Could you check a few things on this model? Use its own coordinates, in mm. A direction names the side the tool comes from. Give positions to 0.01 mm unless a question says otherwise; leave off trailing zeros. Order: outer loops, then holes, each group sorted by start corner. A loop starts at its lowest first (then second) coordinate and runs counter-clockwise, first axis right, second up.
(1) If we mould it in two halves opening along Y, with no side actions, what happens to faces 1 (the flat face through (165.2, -25.6, 67.4)), 2 (the flat face through (107.5, -25, 105)), 3 (the flat face through (142, -150, 82))? For each: released by +Y, released by -Y, zero draft, split by the parting line, or undercut.
(2) Imagine slicing it at D-D, the plane y = -124. Write out the boundary of the cut face in (x, z), then the cut area to 3 significant figures.
(3) Imagine slicing it at A-A, the plane x = 170.5. Write out the boundary of the cut face in (y, z).
(4) On a 3-axis mill with a long thin cutter (end or side, diameter ignored), from which of +Z, -Z, +X, -X, +Y, -Y can I reach the whole of each face in a straight line? I mean faces 4 (the flat face through (99, -60, 20)), 5 (the flat face through (99, 10, 20)), 6 (the flat face through (180, -26, 40)), 7 (the flat face through (65, -26, 83)). Say none if no direction works.
(5) Imagine slicing it at B-B, the plane y = -25. Write out the boundary of the cut face in (x, z).
(6) If I drill on probe 1 along X at (y, z) = (-64.5, 88); probe 2 along Y at (x, z) = (105, 112); probe 3 along Y at (x, z) = (28, 22), over which ranges is the centre line in solid material (lowest first)?
(7) Will these pins go through, and if not, where does the flat tip stop? pin 1 (10 mm diameter, centred on x = 134, z = 11.5, fed in from -Y); pin 2 (2 mm diameter, centred on x = 78.5, z = 69.5, fed in from -Y); pin 3 (12 mm diameter, centred on x = 152, z = 61, fed in from +Y); pin 4 (22 mm diameter, centred on x = 83.5, y = 8.5, fed in from -Z).
(8) Imagine slicing it at C-C, the plane z = 96.5. Write out the boundary of the cut face in (x, y).
from build123d import *

# Parameters (mm, degrees)
SKETCH_1_W          = 200
SKETCH_1_H          = 50
EXTRUDE_1_DEPTH     = 20
SKETCH_2_W          = 160
SKETCH_2_H          = 90
EXTRUDE_2_DEPTH     = 40
SKETCH_3_W          = 15
SKETCH_3_H          = 15
EXTRUDE_3_DEPTH     = 90
EXTRUDE_START       = -45
SKETCH_5_W          = 15
SKETCH_5_H          = 15
EXTRUDE_4_DEPTH     = 125
SKETCH_6_R          = 30
EXTRUDE_5_DEPTH     = 30
SKETCH_7_W          = 30
SKETCH_7_H          = 5
CUT_EXTRUDE_2_DEPTH = 30


with BuildPart() as part:
    # Эскиз1 → Бобышка-Вытянуть1 (new body)
    with BuildSketch(Plane.XY):
        with Locations((100, -25)):
            Rectangle(SKETCH_1_W, SKETCH_1_H)
    extrude(amount=EXTRUDE_1_DEPTH)

    # Эскиз2 → Бобышка-Вытянуть2 (add)
    with BuildSketch(Plane.XY.offset(20)):
        with Locations((100, -25)):
            Rectangle(SKETCH_2_W, SKETCH_2_H)
    extrude(amount=EXTRUDE_2_DEPTH)

    # Эскиз3 → Бобышка-Вытянуть3 (add)
    with BuildSketch(Plane.XZ.offset(70)):
        Polygon((65, 90), (65, 75), (65, 60), (135, 60), (135, 75), (135, 90), align=None)
        with Locations((142.5, 82.5)):
            Rectangle(SKETCH_3_W, SKETCH_3_H)
        Polygon((135, 75), (135, 60), (180, 60), (150, 75), align=None)
        Polygon((65, 75), (20, 60), (65, 60), align=None)
    extrude(amount=-EXTRUDE_3_DEPTH)

    # Эскиз5 → Бобышка-Вытянуть4 (add, symmetric)
    with BuildSketch(Plane(origin=(0, 20, 0), x_dir=(1, 0, 0), z_dir=(0, 1, 0)).offset(EXTRUDE_START)):
        with Locations((142.5, -82.5)):
            Rectangle(SKETCH_5_W, SKETCH_5_H)
    extrude(amount=EXTRUDE_4_DEPTH, both=True)

    # Эскиз6 → Бобышка-Вытянуть5 (add)
    with BuildSketch(Plane.XY.offset(90)):
        with Locations((107.5, -25)):
            Circle(SKETCH_6_R)
    extrude(amount=EXTRUDE_5_DEPTH)

    # Эскиз7 → Вырез-Вытянуть2 (cut)
    with BuildSketch(Plane.XY.offset(120)):
        with Locations((92.5, -27.5)):
            Rectangle(SKETCH_7_W, SKETCH_7_H)
        with Locations((92.5, -22.5)):
            Rectangle(SKETCH_7_W, SKETCH_7_H)
    extrude(amount=-CUT_EXTRUDE_2_DEPTH, mode=Mode.SUBTRACT)


solid = part.part
Answer block:
1. face 1: zero draft
1. face 2: undercut
1. face 3: released by -Y
2. outline: (135, 75) - (150, 75) - (150, 90) - (135, 90) - close
2. area: 225 mm2
3. outline: (-70, 20) - (-50, 20) - (-50, 0) - (0, 0) - (0, 20) - (20, 20) - (20, 64.75) - (-70, 64.75) - close
4. face 4: -Z, +X, -X, -Y
4. face 5: -Z, +X, -X, +Y
4. face 6: +Z, +X, +Y, -Y
4. face 7: +Z, -X, +Y, -Y
5. outline: (0, 0) - (200, 0) - (200, 20) - (180, 20) - (180, 60) - (150, 75) - (150, 90) - (137.5, 90) - (137.5, 120) - (107.5, 120) - (107.5, 90) - (65, 90) - (65, 75) - (20, 60) - (20, 20) - (0, 20) - close
6. probe 1: x = 65 to 150
6. probe 2: y = -54.9 to -30, -20 to 4.9
6. probe 3: y = -70 to 20
7. pin 1: stops at y = -50
7. pin 2: stops at y = -70
7. pin 3: stops at y = 20
7. pin 4: stops at z = 0
8. outline: (77.92, -30) arc R30 ccw (long way) to (77.92, -20) - (107.5, -20) - (107.5, -30) - close
